Verification items for this drawing (mm, ordinates from the low corner). A direction names the side the tool comes from. Round coordinates to 2 decimals unless told otherwise and drop trailing zeros. Order: outer loops, then holes, each group sorted by start corner. A loop starts at its lowest first (then second) coordinate and runs counter-clockwise, first axis right, second up. Notation, with made-up numbers: M -13,72 L 45,72 A15 cw 45,79 Z; hole C -15.5,70 d9. An arc over 180 degrees is marked long. One line per item, written item: value. Start each with the question number.
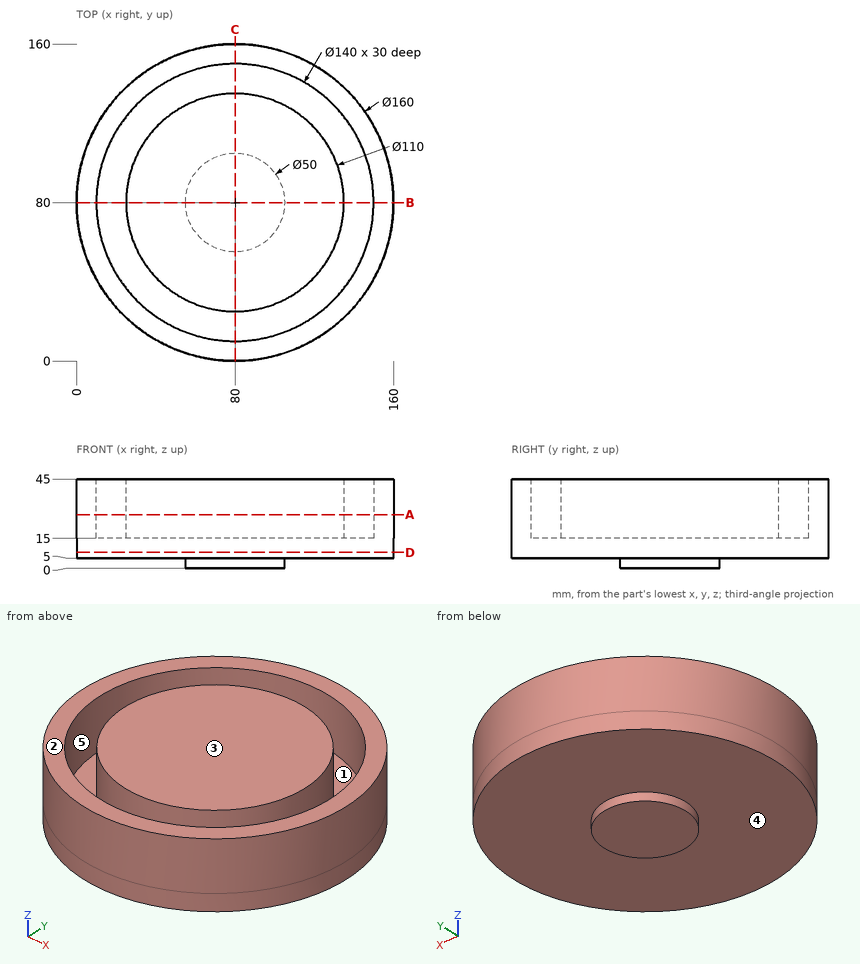
1. Depth check by flat-ended pin: pin 1 (12 mm diameter, centred on x = 96.5, y = 135, fed in from -Z); pin 2 (4 mm diameter, centred on x = 63, z = 25, fed in from -Y); pin 3 (10 mm diameter, centred on x = 91, z = 13.5, fed in from +Y). Enter the tip coordinate at first touch or a pass-through.
2. Section check A-A (z = 27). Record the cut outline in (x, y), and give its area (3 significant figures).
3. Section check B-B (y = 80). Record the cut outline in (x, z), and give its area (3 significant figures).
4. Draft check along X on the marked faces 1 and 2. Enter one of: released by +X, released by -X, zero draft, split by the parting line, or undercut.
5. Scan lines: line 1 along Y through (x, z) = (80, 22.25); line 2 along X through (y, z) = (63.5, 21); line 3 along X through (y, z) = (92.5, 43). Record each from-to range of solid material in increasing order.
6. Section check D-D (z = 8). Record the cut outline in (x, y).
7. Tool access check on the marked faces 3, 4 and 5. Record the directions out of +Z, -Z, +X, -X, +Y, -Y that give a thin tool (end or side, any length) a straight path to the whole face; none if there is none.
Geometry check:
1. pin 1: stops at z = 5
1. pin 2: stops at y = 1.42
1. pin 3: stops at y = 159.77
2. outline: C 80,80 d160; C 80,80 d110; hole C 80,80 d140
2. area: 14,200 mm²
3. outline: M 0,5 L 55,5 L 55,0 L 105,0 L 105,5 L 160,5 L 160,45 L 150,45 L 150,15 L 135,15 L 135,45 L 25,45 L 25,15 L 10,15 L 10,45 L 0,45 Z
3. area: 5,750 mm²
4. face 1: undercut
4. face 2: zero draft
5. line 1: y = 0 to 10, 25 to 135, 150 to 160
5. line 2: x = 1.72 to 11.97, 27.53 to 132.47, 148.03 to 158.28
5. line 3: x = 0.98 to 11.13, 26.44 to 133.56, 148.87 to 159.02
6. outline: C 80,80 d160
7. face 3: +Z, +X, -X, +Y, -Y
7. face 4: -Z
7. face 5: +Z
